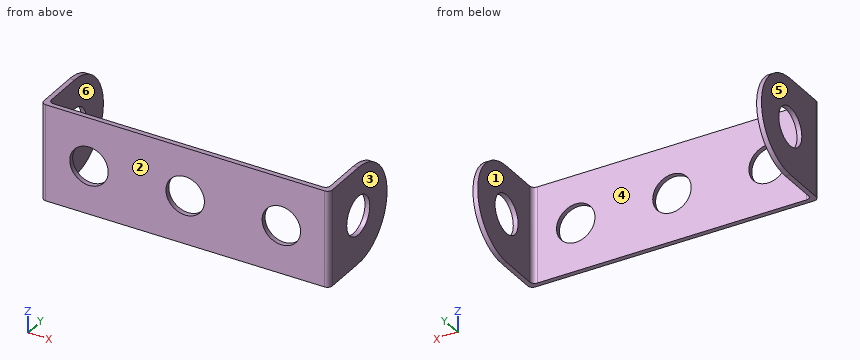
Autodesk Inventor part; units mm, degrees
ref_plane "YZ Plane" through (0, 0, 0) normal (1, 0, 0) x (0, 1, 0)
ref_plane "XZ Plane" through (0, 0, 0) normal (0, 1, 0) x (-1, 0, 0)
ref_plane "XY Plane" through (0, 0, 0) normal (0, 0, 1) x (1, 0, 0)
sketch "Náčrt1" plane through (0, 0, 0) normal (0, 0, 1) x (1, 0, 0)
  line L0 (-14.5, 7.7937) -> (-14.5, -1.7063)
  line L1 (-14.5, -1.7063) -> (14.5, -1.7063)
  line L2 (14.5, -1.7063) -> (14.5, 7.7937)
  line L3 (14.5, 7.7937) -> (15, 7.7937)
  line L4 (15, 7.7937) -> (15, -2.2063)
  line L5 (15, -2.2063) -> (-15, -2.2063)
  line L6 (-15, -2.2063) -> (-15, 7.7937)
  line L7 (-15, 7.7937) -> (-14.5, 7.7937)
  point P0 (0, 0)
  point P1 (14.5, 3.0437)
  point P2 (-14.75, 7.7937)
  point P3 (14.75, 7.7937)
  dimension "d0" = 15
  dimension "d1" = 15
  dimension "d2" = 0.5
  dimension "d3" = 0.5
  dimension "d4" = 0.5
  dimension "d5" = 10
  dimension "d6" = 10
extrude "Vysunutí1" add sketch "Náčrt1" along normal blind 10
sketch "Náčrt2" plane through (15, -2.2063, 0) normal (1, 0, 0) x (0, 0, -1)
  circle A0 centre (-5, 5) radius 2
  line L0 (0, 0) -> (0, 10)
  point P0 (0, 2.2063)
  point P1 (0, 5)
  dimension "d9" = 4
  dimension "d10" = 5
extrude "Vysunutí2" cut sketch "Náčrt2" against normal through all
pattern_linear "Obdélníkové pole1" count 10 spacing 10 along (0, 0, 1) of "Vysunutí2"
sketch "Náčrt3" plane through (-14.5, -1.7063, 0) normal (0, 1, 0) x (1, 0, 0)
  circle A0 centre (4.5, -5) radius 2
  line L0 (29, -10) -> (0, -10)
  line L1 (-0.5, 0) -> (-0.5, -10)
  point P0 (14.5, 0)
  dimension "d16" = 4
  dimension "d17" = 5
  dimension "d18" = 5
extrude "Vysunutí3" cut sketch "Náčrt3" against normal through all
pattern_linear "Obdélníkové pole2" count 10 spacing 10 along (0, 0, -1) count 5 spacing 10 along (1, 0, 0) of "Vysunutí3"
sketch "Náčrt4" plane through (15, -2.2063, 0) normal (1, 0, 0) x (0, 0, -1)
  arc A0 (0, 5) -> (-10, 5) centre (-5, 5) ccw
  line L0 (0, 0) -> (0, 10)
  line L1 (0, 0) -> (-10, 0)
  line L2 (0, 10) -> (-10, 10)
  line L3 (-10, 10) -> (0, 10)
  line L4 (0, 10) -> (0, 5)
  line L5 (0, 10) -> (0, 0.5)
  line L6 (-10, 10) -> (-10, 0.5)
  line L7 (-10, 5) -> (-10, 10)
  point P0 (0, 2.2063)
  point P1 (-5, 10)
  dimension "d27" = 10
  dimension "d28" = 5
  dimension "d29" = 5
extrude "Vysunutí4" cut sketch "Náčrt4" against normal through all
fillet "Zaoblení1" radius 0.5 2 edges at (15, -2.2063, 5) (14.5, -1.7063, 5)
fillet "Zaoblení2" radius 0.5 2 edges at (-15, -2.2063, 5) (-14.5, -1.7063, 5)
properties part number "3031"
Work out the finished part from the listing and answer in its coordinate system (mm). Face numbers are marked on the shaded views. A direction names the side the tool comes from. Give positions to 0.01 mm unless a question says otherwise; leave off trailing zeros. Order: outer loops, then holes, each group sorted by start corner. A loop starts at its lowest first (then second) coordinate and runs counter-clockwise, first axis right, second up. Notation, with made-up numbers: (59.5, -38) -> (69.5, -38) arc R17 cw to (69.5, -5) -> close; hole circle Ø3 at (-3.75, -8). An arc over 180 degrees is marked (long way). Answer as a JSON object with one key per item and string values. Group by question number.
1. Section C-C on z = 5 is taken. Count the separate pieces of the cut face and the enclosed holes in it, plus the area to 3 significant figures.
2. A flat-ended cylindrical pin translates along its axis: pin 1 Ø5 at (x, z) = (-10, 5) entering from +Y. Find the tip coordinate at first contact, or state that the pin passes through.
3. Section D-D on y = 1.75 is taken. Determine the outline of the cut face in (x, z), plus the area to 3 significant figures.
4. Section B-B on x = 10 is taken. Determine the outline of the cut face in (y, z), plus the area to 3 significant figures.
5. The mould has two halves that part along X. Classify the marked faces 1, 2, 3 and 4: released by +X, released by -X, zero draft, split by the parting line, or undercut.
6. Consider line 1 along Z through (x, y) = (0, -2); line 2 along X through (y, z) = (0.25, 8); line 3 along Y through (x, z) = (12.5, 7.5). Determine where each line is inside the solid, lowest interval first. Write a range as [from, to].
7. Section A-A on y = -0.25 is taken. Determine the outline of the cut face in (x, z).
8. A tool of negligible diameter and unlimited length cuts with its end or side. For the marked faces 5 and 6, from which of +Z, -Z, +X, -X, +Y, -Y can it reach the whole face along a straight path? Write none if from no direction.
Result sheet:
{
 "1": {"separate pieces": "6", "enclosed holes": "0", "area": "14.5 mm^2"},
 "2": {"pin 1": "stops at y = -1.71"},
 "3": {"outline": "(-15, 0) -> (-14.5, 0) -> (-14.5, 3.29) -> (-15, 3.29) -> close; (-15, 6.71) -> (-14.5, 6.71) -> (-14.5, 10) -> (-15, 10) -> close; (14.5, 0) -> (15, 0) -> (15, 3.29) -> (14.5, 3.29) -> close; (14.5, 6.71) -> (15, 6.71) -> (15, 10) -> (14.5, 10) -> close", "area": "6.59 mm^2"},
 "4": {"outline": "(-2.21, 0) -> (-1.71, 0) -> (-1.71, 3) -> (-2.21, 3) -> close; (-2.21, 7) -> (-1.71, 7) -> (-1.71, 10) -> (-2.21, 10) -> close", "area": "3.00 mm^2"},
 "5": {"face 1": "undercut", "face 2": "zero draft", "face 3": "released by +X", "face 4": "undercut"},
 "6": {"line 1": "z = [0, 3], [7, 10]", "line 2": "x = [-15, -14.5], [14.5, 15]", "line 3": "y = [-2.21, -1.71]"},
 "7": {"outline": "(-15, 0) -> (-14.5, 0) -> (-14.5, 10) -> (-15, 10) -> close; (14.5, 0) -> (15, 0) -> (15, 10) -> (14.5, 10) -> close"},
 "8": {"face 5": "+Z, -Z, -X, +Y, -Y", "face 6": "+Z, -Z, +Y"}
}
